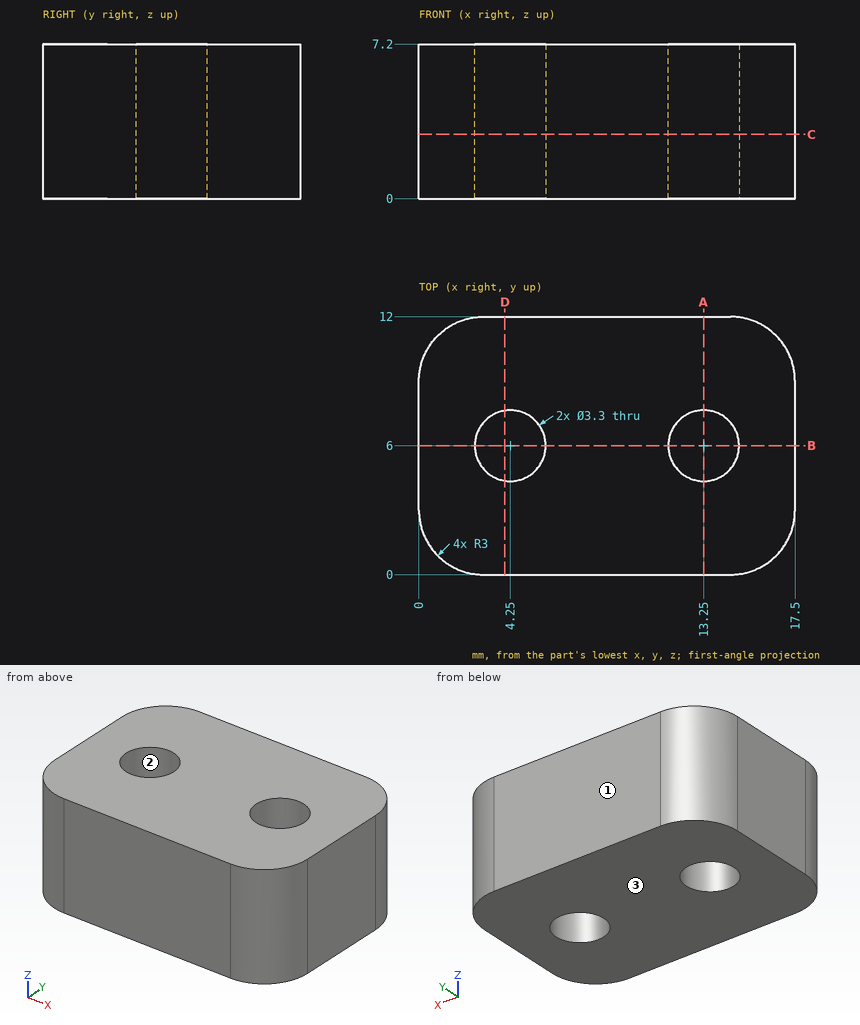
Input: dimensioned drawing with shaded views. Units: mm. Origin: part minimum x, y, z. Round coordinates to 2 decimals unless told otherwise and drop trailing zeros. Loops run counter-clockwise (first coordinate to the right, second up) from the corner with the lowest first, then second, coordinate; pieces in that order, holes last. Notation, with made-up numbers: M -39.75,-5.75 L 18.25,-5.75 A25 cw 18.25,19.25 Z; hole C 84,1 d5. An arc over 180 degrees is marked long. Answer in a Markdown table with one row per item. Add a question column.
1. Mould query, pull axis Y, two halves, no side actions, for the marked faces 1, 2 and 3. Classes: released by +Y, released by -Y, zero draft, split by the parting line, or undercut.
2. Ray query, probe 1 along Y at (x, z) = (4.25, 3.5); probe 2 along Y at (x, z) = (3, 2.5); probe 3 along Y at (x, z) = (2.5, 5.25). Return the intervals inside material, ascending.
3. Contact query for flat-ended pins moving along their axis: pin 1 (3 mm diameter, centred on x = 12, z = 1, fed in from -Y); pin 2 (3 mm diameter, centred on x = 4.25, y = 6, fed in from +Z). Output: stop coordinate, or through.
4. Section B-B (y = 6). Output: boundary loops of the cut face in (x, z), and give its area (3 significant figures).
5. Section C-C (z = 3). Output: boundary loops of the cut face in (x, y), and give its area (3 significant figures).
6. Section D-D (x = 4). Output: boundary loops of the cut face in (y, z).
7. Section A-A (x = 13.25). Output: boundary loops of the cut face in (y, z), and give its area (3 significant figures).
Values follow:
| question | item | result |
|---|---|---|
| 1 | face 1 | released by +Y |
| 1 | face 2 | undercut |
| 1 | face 3 | zero draft |
| 2 | probe 1 | 0 to 4.35, 7.65 to 12 |
| 2 | probe 2 | 0 to 4.92, 7.08 to 12 |
| 2 | probe 3 | 0.04 to 11.96 |
| 3 | pin 1 | y = 0 |
| 3 | pin 2 | through |
| 4 | outline | M 0,0 L 2.6,0 L 2.6,7.2 L 0,7.2 Z; M 5.9,0 L 11.6,0 L 11.6,7.2 L 5.9,7.2 Z; M 14.9,0 L 17.5,0 L 17.5,7.2 L 14.9,7.2 Z |
| 4 | area | 78.5 mm^2 |
| 5 | outline | M 0,3 A3 ccw 3,0 L 14.5,0 A3 ccw 17.5,3 L 17.5,9 A3 ccw 14.5,12 L 3,12 A3 ccw 0,9 Z; hole C 4.25,6 d3.3; hole C 13.25,6 d3.3 |
| 5 | area | 185 mm^2 |
| 6 | outline | M 0,0 L 4.37,0 L 4.37,7.2 L 0,7.2 Z; M 7.63,0 L 12,0 L 12,7.2 L 7.63,7.2 Z |
| 7 | outline | M 0,0 L 4.35,0 L 4.35,7.2 L 0,7.2 Z; M 7.65,0 L 12,0 L 12,7.2 L 7.65,7.2 Z |
| 7 | area | 62.6 mm^2 |
